Input: part model. Units: mm. Frame: model coordinates. A direction names the side the tool comes from. Round coordinates to 2 decimals unless told otherwise and drop trailing zeros. Order: outer loops, then holes, each group sorted by start corner. A loop starts at its lowest first (then second) coordinate and runs counter-clockwise, first axis right, second up. Notation, with made-up numbers: (85, 37.25) -> (100, 37.25) arc R5 ccw to (100, 45.25) -> close; hole circle Ø6 at (24, -23.5). An arc over 180 degrees is marked (long way). Use a Markdown table: item, result.
from build123d import *

# Parameters (mm, degrees)
SKETCH1_W           = 135
SKETCH1_H           = 135
SKETCH1_R           = 47.5
BOSS_EXTRUDE1_DEPTH = 3
SKETCH2_R           = 55
SKETCH2_R_2         = 44.5
BOSS_EXTRUDE2_DEPTH = 10


with BuildPart() as part:
    # Sketch1 → Boss-Extrude1 (new body)
    with BuildSketch(Plane(origin=(0, 0, 0), x_dir=(1, 0, 0), z_dir=(0, 1, 0))):
        Rectangle(SKETCH1_W, SKETCH1_H)
        Circle(SKETCH1_R, mode=Mode.SUBTRACT)
    extrude(amount=BOSS_EXTRUDE1_DEPTH)

    # Sketch2 → Boss-Extrude2 (add)
    with BuildSketch(Plane.XZ):
        Circle(SKETCH2_R)
        Circle(SKETCH2_R_2, mode=Mode.SUBTRACT)
    extrude(amount=BOSS_EXTRUDE2_DEPTH)


solid = part.part
1) Cut plane B-B on z = 0. Return loops of the section in (x, y).
Results found:
| item | result |
|---|---|
| outline | (-67.5, 0) -> (-55, 0) -> (-55, -10) -> (-44.5, -10) -> (-44.5, 0) -> (-47.5, 0) -> (-47.5, 3) -> (-67.5, 3) -> close; (44.5, -10) -> (55, -10) -> (55, 0) -> (67.5, 0) -> (67.5, 3) -> (47.5, 3) -> (47.5, 0) -> (44.5, 0) -> close |
2) Set-up query: faces 4 (the cylindrical face through (-10.3, 1.48, 46.37)), 5 (the cylindrical face through (-11.923, -4.93, -53.692)), 6 (the cylindrical face through (-32.798, -4.93, 30.075)). Return all of +Z, -Z, +X, -X, +Y, -Y with unobstructed straight access to the full face (end or side cutting, diameter ignored); none if empty.
Results found:
| item | result |
|---|---|
| face 4 | +Y |
| face 5 | -Y |
| face 6 | +Y, -Y |
3) Line query: L1, parallel to X at y = 2.1, z = 0; L2, parallel to Z at x = 0, y = -8. Output: solid intervals per line, ascending. Write a range as [from, to].
Results found:
| item | result |
|---|---|
| L1 | x = [-67.5, -47.5], [47.5, 67.5] |
| L2 | z = [-55, -44.5], [44.5, 55] |
4) Pull-direction query (Z, two-part tool) for faces 1 (the flat face through (-1, 1, -67.5)), 2 (the flat face through (-31, 0, -46)), 3 (the flat face through (-14.3, 0, 42.4)); classes: +Z half, -Z half, draft (parallel to the pull), parting line (faces both ways), or undercut.
Results found:
| item | result |
|---|---|
| face 1 | -Z half |
| face 2 | draft |
| face 3 | undercut |
5) Cut plane D-D on z = 51. Return loops of the section in (x, y), and give its area (3 significant figures).
Results found:
| item | result |
|---|---|
| outline | (-67.5, 0) -> (-20.59, 0) -> (-20.59, -10) -> (20.59, -10) -> (20.59, 0) -> (67.5, 0) -> (67.5, 3) -> (-67.5, 3) -> close |
| area | 817 mm² |
6) Pin query (flat end, axial travel): pin 1 Ø1.5 at (y, z) = (-7.5, 50) entering from +X; pin 2 Ø4 at (y, z) = (-5, 2) entering from +X; pin 3 Ø2 at (x, y) = (46, -1.5) entering from +Z. Return the tip coordinate at first contact, or that it passes through.
Results found:
| item | result |
|---|---|
| pin 1 | stops at x = 24.48 |
| pin 2 | stops at x = 55 |
| pin 3 | stops at z = 31.62 |
7) Cut plane A-A on x = 0. Return loops of the section in (y, z), and give its area (3 significant figures).
Results found:
| item | result |
|---|---|
| outline | (-10, -55) -> (0, -55) -> (0, -67.5) -> (3, -67.5) -> (3, -47.5) -> (0, -47.5) -> (0, -44.5) -> (-10, -44.5) -> close; (-10, 44.5) -> (0, 44.5) -> (0, 47.5) -> (3, 47.5) -> (3, 67.5) -> (0, 67.5) -> (0, 55) -> (-10, 55) -> close |
| area | 330 mm² |
8) Cut plane C-C on y = -2.25. Return loops of the section in (x, z), and give its area (3 significant figures).
Results found:
| item | result |
|---|---|
| outline | circle Ø110 at (0, 0); hole circle Ø89 at (0, 0) |
| area | 3,280 mm² |
